The listing builds one solid part. Answer for the finished solid, in the listing's coordinates (mm). Face numbers are marked on the shaded views. A direction names the side the tool comes from. Coordinates: 2 decimals unless noted, no trailing zeros. Loops run counter-clockwise (first coordinate to the right, second up) from the corner with the lowest first, then second, coordinate; pieces in that order, holes last. Notation, with made-up numbers: M 18.25,52 L 32.25,52 A4 ccw 32.25,57 Z; hole C 5.5,89 d11. An arc over 180 degrees is marked long. Answer in a Markdown table with one row per item. Add a question column.
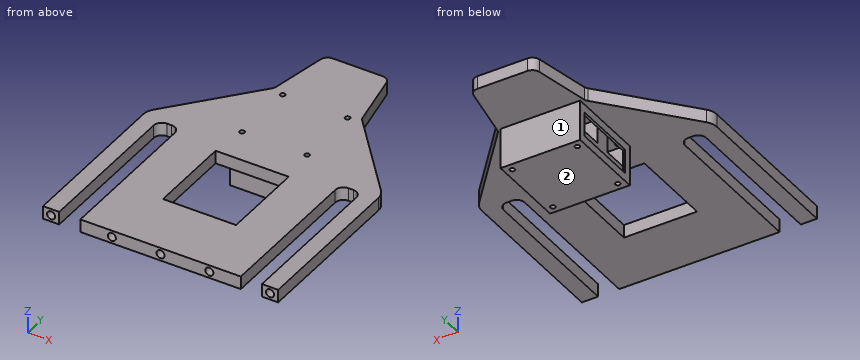
from build123d import *

# Parameters (mm, degrees)
BOSS_EXTRUDE1_DEPTH    = 8
SKETCH2_W              = 45
SKETCH2_H              = 52
CUT_EXTRUDE1_DEPTH     = 342.206659287
SPLIT1_SURFACE_1_BACK  = 343.199
SPLIT1_SURFACE_1_DEPTH = 686.398
SPLIT1_SURFACE_2_BACK  = 343.199
SPLIT1_SURFACE_2_DEPTH = 686.398
SKETCH5_R              = 2.5
CUT_EXTRUDE6_DEPTH     = 5.2
SKETCH4_R              = 2.5
CUT_EXTRUDE7_DEPTH     = 5.2
SKETCH6_R              = 1.5
CUT_EXTRUDE8_DEPTH     = 342.206659287
SKETCH7_W              = 49
SKETCH7_H              = 49
SKETCH7_W_2            = 18
SKETCH7_H_2            = 18
BOSS_EXTRUDE2_DEPTH    = 15
SKETCH8_W              = 49
SKETCH8_H              = 49
SKETCH8_R              = 1.5
BOSS_EXTRUDE3_DEPTH    = 10
SKETCH9_W              = 15
SKETCH9_H              = 40
CUT_EXTRUDE9_DEPTH     = 1.5
SKETCH11_W             = 15
SKETCH11_H             = 40
CUT_EXTRUDE10_DEPTH    = 1.5


with BuildPart() as part:
    # Sketch1 → Boss-Extrude1 (new body)
    with BuildSketch(Plane.XY):
        with BuildLine():
            Line((70, 309.985818768), (85.299227191, 309.985818768))
            ThreePointArc((85.299227191, 309.985818768), (88.489017574, 308.836174247), (90.211957942, 305.915913694))
            Line((90.211957942, 305.915913694), (96.672728921, 271.790334282))
            ThreePointArc((96.672728921, 271.790334282), (97.06575438, 270.906904614), (97.621470019, 270.115641625))
            Line((97.621470019, 270.115641625), (139.950460317, 220.786053348))
            ThreePointArc((139.950460317, 220.786053348), (141.739336996, 217.746026552), (142.361429131, 214.274017901))
            Line((142.361429131, 214.274017901), (142.361429131, 30.859943174))
            ThreePointArc((142.361429131, 30.859943174), (140.896963037, 27.324409268), (137.361429131, 25.859943174))
            Line((137.361429131, 25.859943174), (114.717190871, 25.782318449))
            ThreePointArc((114.717190871, 25.782318449), (112.681998989, 25.341726514), (111.002773989, 24.110332733))
            Line((111.002773989, 24.110332733), (89.38285929, 0))
            Line((89.38285929, 0), (50.5, 0))
            Line((50.5, 0), (28.997226011, 24.110332733))
            ThreePointArc((28.997226011, 24.110332733), (27.318001011, 25.341726514), (25.282809129, 25.782318449))
            Line((25.282809129, 25.782318449), (2.638570869, 25.859943174))
            ThreePointArc((2.638570869, 25.859943174), (-0.896963037, 27.324409268), (-2.361429131, 30.859943174))
            Line((-2.361429131, 30.859943174), (-2.361429131, 214.274017901))
            ThreePointArc((-2.361429131, 214.274017901), (-1.739336996, 217.746026552), (0.049539683, 220.786053348))
            Line((0.049539683, 220.786053348), (42.261389271, 270.115641625))
            ThreePointArc((42.261389271, 270.115641625), (42.81710491, 270.906904614), (43.210130369, 271.790334282))
            Line((43.210130369, 271.790334282), (49.724618218, 305.923183314))
            ThreePointArc((49.724618218, 305.923183314), (51.449026762, 308.838533573), (54.635967087, 309.985818768))
            Line((54.635967087, 309.985818768), (70, 309.985818768))
        make_face()
        with BuildLine():
            Line((7.638570869, 35.492492662), (20.638570869, 35.492492662))
            Line((20.638570869, 35.492492662), (20.638570869, 208.625959477))
            ThreePointArc((20.638570869, 208.625959477), (19.174104775, 212.161493383), (15.638570869, 213.625959477))
            Line((15.638570869, 213.625959477), (12.638570869, 213.625959477))
            ThreePointArc((12.638570869, 213.625959477), (9.103036963, 212.161493383), (7.638570869, 208.625959477))
            Line((7.638570869, 208.625959477), (7.638570869, 35.492492662))
        make_face(mode=Mode.SUBTRACT)
        with BuildLine():
            Line((127.361429131, 35.492492662), (124.361429131, 35.492492662))
            ThreePointArc((124.361429131, 35.492492662), (120.825895225, 36.956958756), (119.361429131, 40.492492662))
            Line((119.361429131, 40.492492662), (119.361429131, 208.625959477))
            ThreePointArc((119.361429131, 208.625959477), (120.825895225, 212.161493383), (124.361429131, 213.625959477))
            Line((124.361429131, 213.625959477), (127.361429131, 213.625959477))
            ThreePointArc((127.361429131, 213.625959477), (130.896963037, 212.161493383), (132.361429131, 208.625959477))
            Line((132.361429131, 208.625959477), (132.361429131, 40.492492662))
            ThreePointArc((132.361429131, 40.492492662), (130.896963037, 36.956958756), (127.361429131, 35.492492662))
        make_face(mode=Mode.SUBTRACT)
    extrude(amount=BOSS_EXTRUDE1_DEPTH)

    # Sketch2 → Cut-Extrude1 (cut, through all)
    with BuildSketch(Plane.XY.offset(8)):
        with Locations((69.88285929, 180.008918923)):
            Rectangle(SKETCH2_W, SKETCH2_H)
    extrude(amount=-CUT_EXTRUDE1_DEPTH, mode=Mode.SUBTRACT)


with BuildPart() as body_2:
    # Split1: the piece behind the surface
    add(part.part)
    # Split1 surface: a surface, the sketch's curves swept straight by 686.398 mm
    with BuildLine(Plane(origin=(0, 0, 0), x_dir=(-1, 0, 0), z_dir=(0, 0, -1)).offset(-SPLIT1_SURFACE_1_BACK), mode=Mode.PRIVATE) as split1_surface_1_path:
        Line((-142.361429131, 115.359943174), (2.361429131, 115.359943174))
    split1_surface_1 = Shell.extrude(split1_surface_1_path.wire(), (0 * SPLIT1_SURFACE_1_DEPTH, 0 * SPLIT1_SURFACE_1_DEPTH, -1 * SPLIT1_SURFACE_1_DEPTH))
    split(bisect_by=split1_surface_1, keep=Keep.BOTTOM)

    # Sketch5 → Cut-Extrude6 (cut)
    with BuildSketch(Plane(origin=(0, 115.359943174, -115.359943174), x_dir=(1, 0, 0), z_dir=(0, -1, 0))):
        with Locations(Location((70, 119.359943174, 0), (0, 0, 270))):
            Circle(SKETCH5_R)
        with Locations(Location((40, 119.359943174, 0), (0, 0, 270))):
            Circle(SKETCH5_R)
        with Locations(Location((2.638570869, 119.359943174, 0), (0, 0, 270))):
            Circle(SKETCH5_R)
    extrude(amount=CUT_EXTRUDE6_DEPTH, mode=Mode.SUBTRACT)


with BuildPart() as part_1:
    add(part.part)

    # Split1: split by a surface, the side it looks to stays
    # Split1 surface: a surface, the sketch's curves swept straight by 686.398 mm
    with BuildLine(Plane(origin=(0, 0, 0), x_dir=(-1, 0, 0), z_dir=(0, 0, -1)).offset(-SPLIT1_SURFACE_2_BACK), mode=Mode.PRIVATE) as split1_surface_2_path:
        Line((-142.361429131, 115.359943174), (2.361429131, 115.359943174))
    split1_surface_2 = Shell.extrude(split1_surface_2_path.wire(), (0 * SPLIT1_SURFACE_2_DEPTH, 0 * SPLIT1_SURFACE_2_DEPTH, -1 * SPLIT1_SURFACE_2_DEPTH))
    split(bisect_by=split1_surface_2, keep=Keep.TOP)

    # Sketch4 → Cut-Extrude7 (cut)
    with BuildSketch(Plane(origin=(0, 115.359943174, 0), x_dir=(-1, 0, 0), z_dir=(0, -1, 0))):
        with Locations(Location((-70, -4, 0), (0, 0, 270))):
            Circle(SKETCH4_R)
        with Locations(Location((-40, -4, 0), (0, 0, 270))):
            Circle(SKETCH4_R)
        with Locations(Location((-100, -4, 0), (0, 0, 270))):
            Circle(SKETCH4_R)
        with Locations(Location((-137.361429131, -4, 0), (0, 0, 90))):
            Circle(SKETCH4_R)
        with Locations(Location((-2.638570869, -4, 0), (0, 0, 270))):
            Circle(SKETCH4_R)
    extrude(amount=-CUT_EXTRUDE7_DEPTH, mode=Mode.SUBTRACT)

    # Sketch6 → Cut-Extrude8 (cut, through all)
    with BuildSketch(Plane.XY.offset(8)):
        with Locations((50.000130369, 267.980334282)):
            Circle(SKETCH6_R)
        with Locations((90.000130369, 267.980334282)):
            Circle(SKETCH6_R)
        with Locations((90.000130369, 227.980334282)):
            Circle(SKETCH6_R)
        with Locations((50.000130369, 227.980334282)):
            Circle(SKETCH6_R)
    extrude(amount=-CUT_EXTRUDE8_DEPTH, mode=Mode.SUBTRACT)

    # Sketch7 → Boss-Extrude2 (add)
    with BuildSketch(Plane(origin=(0, 0, 0), x_dir=(-1, 0, 0), z_dir=(0, 0, -1))):
        with Locations((-70.000130369, 247.980334282)):
            Rectangle(SKETCH7_W, SKETCH7_H)
        with Locations((-56.000130369, 261.980334282)):
            Rectangle(SKETCH7_W_2, SKETCH7_H_2, mode=Mode.SUBTRACT)
        with Locations((-84.000130369, 261.980334282)):
            Rectangle(SKETCH7_W_2, SKETCH7_H_2, mode=Mode.SUBTRACT)
        with Locations((-84.000130369, 233.980334282)):
            Rectangle(SKETCH7_W_2, SKETCH7_H_2, mode=Mode.SUBTRACT)
        with Locations((-56.000130369, 233.980334282)):
            Rectangle(SKETCH7_W_2, SKETCH7_H_2, mode=Mode.SUBTRACT)
    extrude(amount=BOSS_EXTRUDE2_DEPTH)

    # Sketch8 → Boss-Extrude3 (add)
    with BuildSketch(Plane(origin=(0, 0, -15), x_dir=(-1, 0, 0), z_dir=(0, 0, -1))):
        with Locations((-70.000130369, 247.980334282)):
            Rectangle(SKETCH8_W, SKETCH8_H)
        with Locations(Location((-50.000130369, 267.980334282, 0), (0, 0, 180))):
            Circle(SKETCH8_R, mode=Mode.SUBTRACT)
        with Locations(Location((-90.000130369, 267.980334282, 0), (0, 0, 180))):
            Circle(SKETCH8_R, mode=Mode.SUBTRACT)
        with Locations(Location((-50.000130369, 227.980334282, 0), (0, 0, 180))):
            Circle(SKETCH8_R, mode=Mode.SUBTRACT)
        with Locations(Location((-90.000130369, 227.980334282, 0), (0, 0, 180))):
            Circle(SKETCH8_R, mode=Mode.SUBTRACT)
    extrude(amount=BOSS_EXTRUDE3_DEPTH)

    # Sketch9 → Cut-Extrude9 (cut)
    with BuildSketch(Plane.ZY.offset(-45.500130369)):
        with Locations((-12.5, 247.980334282)):
            Rectangle(SKETCH9_W, SKETCH9_H)
    extrude(amount=-CUT_EXTRUDE9_DEPTH, mode=Mode.SUBTRACT)

    # Sketch11 → Cut-Extrude10 (cut)
    with BuildSketch(Plane(origin=(94.500130369, 0, 0), x_dir=(0, 0, -1), z_dir=(1, 0, 0))):
        with Locations((12.5, 247.980334282)):
            Rectangle(SKETCH11_W, SKETCH11_H)
    extrude(amount=-CUT_EXTRUDE10_DEPTH, mode=Mode.SUBTRACT)


solid = part_1.part
(1) A cutting plane is placed at C-C (z = 4). State how many separate pieces and enclosed holes the cut face has, plus the area to 3 significant figures.
(2) A cutting plane is placed at B-B (y = 193.5). Give the vertices of the cut face in (x, z).
(3) A cutting plane is placed at D-D (z = -10.5). Give the vertices of the cut face in (x, y), plus the area to 3 significant figures.
(4) A cutting plane is placed at A-A (x = 78.5). Give the vertices of the cut face in (y, z).
(5) Each of these flat-tipped pins is pushed along its axis until it touches: pin 1 (6 mm diameter, centred on x = 36.5, z = -1.5, fed in from +Y); pin 2 (1.5 mm diameter, centred on x = 101, z = 5, fed in from -Y); pin 3 (7.5 mm diameter, centred on y = 264.5, z = -4, fed in from +X); pin 4 (2.5 mm diameter, centred on x = 90, y = 227.98, fed in from +Z). Where does it stop, or does it pass through?
(6) Straight lines are drawn through the part: line 1 (X direction, y = 269, z = -7); line 2 (X direction, y = 195, z = 0.5); line 3 (Y direction, x = 59.5, z = -1.5). For each, find the intervals that lie inside material, in ascending order.
(7) For the marked faces 1 and 2, determine the directions among +Z, -Z, +X, -X, +Y, -Y from which every point of the face is accessible in a straight line to the end or side of a thin tool.
Solved:
| question | item | result |
|---|---|---|
| 1 | separate pieces | 1 |
| 1 | enclosed holes | 5 |
| 1 | area | 16,900 mm² |
| 2 | outline | M -2.36,0 L 7.64,0 L 7.64,8 L -2.36,8 Z; M 20.64,0 L 47.38,0 L 47.38,8 L 20.64,8 Z; M 92.38,0 L 119.36,0 L 119.36,8 L 92.38,8 Z; M 132.36,0 L 142.36,0 L 142.36,8 L 132.36,8 Z |
| 3 | outline | M 45.5,223.48 L 94.5,223.48 L 94.5,227.98 L 93,227.98 L 93,224.98 L 75,224.98 L 75,242.98 L 93,242.98 L 93,252.98 L 75,252.98 L 75,270.98 L 93,270.98 L 93,267.98 L 94.5,267.98 L 94.5,272.48 L 45.5,272.48 L 45.5,267.98 L 47,267.98 L 47,270.98 L 65,270.98 L 65,252.98 L 47,252.98 L 47,242.98 L 65,242.98 L 65,224.98 L 47,224.98 L 47,227.98 L 45.5,227.98 Z |
| 3 | area | 985 mm² |
| 4 | outline | M 115.36,0 L 154.01,0 L 154.01,8 L 115.36,8 Z; M 206.01,0 L 223.48,0 L 223.48,-25 L 272.48,-25 L 272.48,0 L 309.99,0 L 309.99,8 L 206.01,8 Z; hole M 224.98,-15 L 242.98,-15 L 242.98,0 L 224.98,0 Z; hole M 252.98,-15 L 270.98,-15 L 270.98,0 L 252.98,0 Z |
| 5 | pin 1 | stops at y = 266.42 |
| 5 | pin 2 | stops at y = 120.56 |
| 5 | pin 3 | stops at x = 94.5 |
| 5 | pin 4 | passes through |
| 6 | line 1 | x = 45.5 to 47, 65 to 75, 93 to 94.5 |
| 6 | line 2 | x = -2.36 to 7.64, 20.64 to 47.38, 92.38 to 119.36, 132.36 to 142.36 |
| 6 | line 3 | y = 223.48 to 224.98, 242.98 to 252.98, 270.98 to 272.48 |
| 7 | face 1 | -Z, +X, -X, +Y |
| 7 | face 2 | -Z, +X, -X, +Y, -Y |
